```python
from build123d import *

# Parameters (mm, degrees)
DODANIE_WYCI_GNI_CIE1_DEPTH = 5
DODANIE_WYCI_GNI_CIE4_DEPTH = 8
DODANIE_WYCI_GNI_CIE5_DEPTH = 3
SZKIC8_R                    = 1.05
WYTNIJ_WYCI_GNI_CIE1_DEPTH  = 38.825793195
SZKIC9_R                    = 1.05
WYTNIJ_WYCI_GNI_CIE2_DEPTH  = 39.000906522
ZAOKR_GLENIE1_R             = 2.5
ZAOKR_GLENIE2_R             = 2.5
ZAOKR_GLENIE3_R             = 2
WYTNIJ_WYCI_GNI_CIE3_DEPTH  = 38.825793195


# Some blends are built 0.0001 mm under size
with BuildPart() as part:
    # Szkic1 → Dodanie-wyciągnięcie1 (new body)
    with BuildSketch(Plane.XY):
        Polygon((6.943729276, -9.167385079), (6.943729276, -12.167385079), (-29.356270724, -12.167385079), (-29.356270724, -9.167385079), (-26.62744343, -9.167385079), (-26.62744343, 10.832614921), (-23.706270724, 10.832614921), (-23.706270724, -9.167385079), (1.293729276, -9.167385079), (1.293729276, 10.832614921), (4.214901981, 10.832614921), (4.214901981, -9.167385079), align=None)
    extrude(amount=DODANIE_WYCI_GNI_CIE1_DEPTH)

    # Szkic5 → Dodanie-wyciągnięcie4 (add)
    with BuildSketch(Plane.XY.offset(5)):
        Polygon((-26.62744343, -9.167385079), (-23.706270724, -9.167385079), (1.293729276, -9.167385079), (4.214901981, -9.167385079), (6.943729276, -9.167385079), (6.943729276, -12.167385079), (-29.356270724, -12.167385079), (-29.356270724, -9.167385079), align=None)
    extrude(amount=DODANIE_WYCI_GNI_CIE4_DEPTH)

    # Szkic7 → Dodanie-wyciągnięcie5 (add)
    with BuildSketch(Plane(origin=(0, 0, 0), x_dir=(-1, 0, 0), z_dir=(0, 0, -1))):
        Polygon((-4.214901981, -9.167385079), (-1.293729276, -9.167385079), (23.706270724, -9.167385079), (26.62744343, -9.167385079), (29.356270724, -9.167385079), (29.356270724, -12.167385079), (-6.943729276, -12.167385079), (-6.943729276, -9.167385079), align=None)
    extrude(amount=DODANIE_WYCI_GNI_CIE5_DEPTH)

    # Szkic8 → Wytnij-wyciągnięcie1 (cut, through all)
    with BuildSketch(Plane(origin=(0, -9.167385079, 0), x_dir=(1, 0, 0), z_dir=(0, 1, 0))):
        with Locations(Location((4.446418634, -8, 0), (0, 0, 180))):
            Circle(SZKIC8_R)
        with Locations(Location((-26.853581366, -8, 0), (0, 0, 180))):
            Circle(SZKIC8_R)
    extrude(amount=-WYTNIJ_WYCI_GNI_CIE1_DEPTH, mode=Mode.SUBTRACT)

    # Szkic9 → Wytnij-wyciągnięcie2 (cut, through all)
    with BuildSketch(Plane.ZY.offset(26.62744343)):
        with Locations((2.5, 8.332614921)):
            Circle(SZKIC9_R)
    extrude(amount=-WYTNIJ_WYCI_GNI_CIE2_DEPTH, mode=Mode.SUBTRACT)

    # Zaokrąglenie1
    zaokr_glenie1_edges = [part.edges().sort_by_distance(p)[0] for p in [
        (-29.356270724, -10.667385079, 13),
        (6.943729276, -10.667385079, 13),
        (6.943729276, -10.667385079, -3),
        (-29.356270724, -10.667385079, -3),
    ]]
    fillet(zaokr_glenie1_edges, radius=ZAOKR_GLENIE1_R)

    # Zaokrąglenie2
    zaokr_glenie2_edges = [part.edges().sort_by_distance(p)[0] for p in [
        (-25.166857077, 10.832614921, 5),
        (-25.166857077, 10.832614921, 0),
        (2.754315628, 10.832614921, 5),
        (2.754315628, 10.832614921, 0),
    ]]
    fillet(zaokr_glenie2_edges, radius=ZAOKR_GLENIE2_R - 0.0001)  # a hair under: the kernel refuses the full size

    # Zaokrąglenie3
    # the kernel refuses this fillet: 2 mm, written as the material it adds along each edge
    with BuildSketch(Plane(origin=(4.214901981, -9.167385079, 0), x_dir=(1, 0, 0), z_dir=(0, 0, 1))) as zaokr_glenie3_piece_1:
        with BuildLine():
            CenterArc((ZAOKR_GLENIE3_R, ZAOKR_GLENIE3_R), ZAOKR_GLENIE3_R, 180, 90)
            Line((0, ZAOKR_GLENIE3_R), (0, 0))
            Line((0, 0), (ZAOKR_GLENIE3_R, 0))
        make_face()
    extrude(amount=5)
    with BuildSketch(Plane(origin=(-26.62744343, -9.167385079, 0), x_dir=(-1, 0, 0), z_dir=(0, 0, 1))) as zaokr_glenie3_piece_2:
        with BuildLine():
            CenterArc((ZAOKR_GLENIE3_R, -ZAOKR_GLENIE3_R), ZAOKR_GLENIE3_R, 90, 90)
            Line((0, -ZAOKR_GLENIE3_R), (0, 0))
            Line((0, 0), (ZAOKR_GLENIE3_R, 0))
        make_face()
    extrude(amount=5)
    with BuildSketch(Plane(origin=(-23.706270724, -9.167385079, 5), x_dir=(0, 1, 0), z_dir=(-1, 0, 0))) as zaokr_glenie3_piece_3_section:
        with BuildLine():
            CenterArc((ZAOKR_GLENIE3_R, -ZAOKR_GLENIE3_R), ZAOKR_GLENIE3_R, 90, 90)
            Line((0, -ZAOKR_GLENIE3_R), (0, 0))
            Line((0, 0), (ZAOKR_GLENIE3_R, 0))
        make_face()
    zaokr_glenie3_piece_3 = extrude(amount=2.921172706, mode=Mode.PRIVATE)
    zaokr_glenie3_piece_3 = zaokr_glenie3_piece_3 - Plane(origin=(-26.853581366, -8.714586813, 8), x_dir=(-1, 0, 0), z_dir=(0, 1, 0)) * Cylinder(1.05, 14, mode=Mode.PRIVATE)
    add(zaokr_glenie3_piece_3)
    with BuildSketch(Plane(origin=(4.214901981, -9.167385079, 5), x_dir=(0, 0, 1), z_dir=(-1, 0, 0))) as zaokr_glenie3_piece_4_section:
        with BuildLine():
            CenterArc((ZAOKR_GLENIE3_R, ZAOKR_GLENIE3_R), ZAOKR_GLENIE3_R, 180, 90)
            Line((0, ZAOKR_GLENIE3_R), (0, 0))
            Line((0, 0), (ZAOKR_GLENIE3_R, 0))
        make_face()
    zaokr_glenie3_piece_4 = extrude(amount=2.921172706, mode=Mode.PRIVATE)
    zaokr_glenie3_piece_4 = zaokr_glenie3_piece_4 - Plane(origin=(4.446418634, -8.714587659, 8), x_dir=(-1, 0, 0), z_dir=(0, 1, 0)) * Cylinder(1.05, 14, mode=Mode.PRIVATE)
    add(zaokr_glenie3_piece_4)
    with BuildSketch(Plane(origin=(1.293729276, -9.167385079, 0), x_dir=(0, 0, -1), z_dir=(1, 0, 0))) as zaokr_glenie3_piece_5:
        with BuildLine():
            CenterArc((ZAOKR_GLENIE3_R, ZAOKR_GLENIE3_R), ZAOKR_GLENIE3_R, 180, 90)
            Line((0, ZAOKR_GLENIE3_R), (0, 0))
            Line((0, 0), (ZAOKR_GLENIE3_R, 0))
        make_face()
    extrude(amount=2.921172706)
    with BuildSketch(Plane(origin=(-26.62744343, -9.167385079, 0), x_dir=(0, 1, 0), z_dir=(1, 0, 0))) as zaokr_glenie3_piece_6:
        with BuildLine():
            CenterArc((ZAOKR_GLENIE3_R, -ZAOKR_GLENIE3_R), ZAOKR_GLENIE3_R, 90, 90)
            Line((0, -ZAOKR_GLENIE3_R), (0, 0))
            Line((0, 0), (ZAOKR_GLENIE3_R, 0))
        make_face()
    extrude(amount=2.921172706)
    with BuildSketch(Plane(origin=(4.214901981, -9.167385079, -5), x_dir=(1, 0, 0), z_dir=(0, 0, 1))) as zaokr_glenie3_piece_7a_section:
        with BuildLine():
            CenterArc((ZAOKR_GLENIE3_R, ZAOKR_GLENIE3_R), ZAOKR_GLENIE3_R, 180, 90)
            Line((0, ZAOKR_GLENIE3_R), (0, 0))
            Line((0, 0), (ZAOKR_GLENIE3_R, 0))
        make_face()
    zaokr_glenie3_piece_7a = extrude(amount=10, mode=Mode.PRIVATE)
    zaokr_glenie3_piece_7a = zaokr_glenie3_piece_7a & Plane(origin=(4.443729276, -8.70886388, -0.5), x_dir=(1, 0, 0), z_dir=(0, 1, 0)) * Cylinder(2.5, 28, mode=Mode.PRIVATE)
    zaokr_glenie3_piece_7a = split(zaokr_glenie3_piece_7a, bisect_by=Plane(origin=(4.654982767, -8.70886388, 0), z_dir=(0, 0, -1)), keep=Keep.TOP, mode=Mode.PRIVATE)
    with BuildSketch(Plane(origin=(1.293729276, -9.167385079, 0), x_dir=(0, 0, -1), z_dir=(1, 0, 0))) as zaokr_glenie3_piece_7b_section:
        with BuildLine():
            CenterArc((ZAOKR_GLENIE3_R, ZAOKR_GLENIE3_R), ZAOKR_GLENIE3_R, 180, 90)
            Line((0, ZAOKR_GLENIE3_R), (0, 0))
            Line((0, 0), (ZAOKR_GLENIE3_R, 0))
        make_face()
    zaokr_glenie3_piece_7b = extrude(amount=7.921172706, mode=Mode.PRIVATE)
    zaokr_glenie3_piece_7b = zaokr_glenie3_piece_7b & Plane(origin=(4.443729276, -8.713013539, -0.5), x_dir=(1, 0, 0), z_dir=(0, 1, 0)) * Cylinder(2.5, 24, mode=Mode.PRIVATE)
    zaokr_glenie3_piece_7b = split(zaokr_glenie3_piece_7b, bisect_by=Plane(origin=(4.214901981, -8.713013539, -0.447003407), z_dir=(1, 0, 0)), keep=Keep.TOP, mode=Mode.PRIVATE)
    zaokr_glenie3_piece_7 = zaokr_glenie3_piece_7a & zaokr_glenie3_piece_7b
    add(zaokr_glenie3_piece_7)
    with BuildSketch(Plane(origin=(4.214901981, -9.167385079, 0), x_dir=(1, 0, 0), z_dir=(0, 0, 1))) as zaokr_glenie3_piece_8a_section:
        with BuildLine():
            CenterArc((ZAOKR_GLENIE3_R, ZAOKR_GLENIE3_R), ZAOKR_GLENIE3_R, 180, 90)
            Line((0, ZAOKR_GLENIE3_R), (0, 0))
            Line((0, 0), (ZAOKR_GLENIE3_R, 0))
        make_face()
    zaokr_glenie3_piece_8a = extrude(amount=10, mode=Mode.PRIVATE)
    zaokr_glenie3_piece_8a = zaokr_glenie3_piece_8a - Plane(origin=(4.446418634, -9.113524986, 8), x_dir=(-1, 0, 0), z_dir=(0, 1, 0)) * Cylinder(1.05, 28, mode=Mode.PRIVATE)
    zaokr_glenie3_piece_8a = split(zaokr_glenie3_piece_8a, bisect_by=Plane(origin=(5.693435365, -9.113524986, 5), z_dir=(0, 0, 1)), keep=Keep.TOP, mode=Mode.PRIVATE)
    with BuildSketch(Plane(origin=(9.214901981, -9.167385079, 5), x_dir=(0, 0, 1), z_dir=(-1, 0, 0))) as zaokr_glenie3_piece_8b_section:
        with BuildLine():
            CenterArc((ZAOKR_GLENIE3_R, ZAOKR_GLENIE3_R), ZAOKR_GLENIE3_R, 180, 90)
            Line((0, ZAOKR_GLENIE3_R), (0, 0))
            Line((0, 0), (ZAOKR_GLENIE3_R, 0))
        make_face()
    zaokr_glenie3_piece_8b = extrude(amount=7.921172706, mode=Mode.PRIVATE)
    zaokr_glenie3_piece_8b = split(zaokr_glenie3_piece_8b, bisect_by=Plane(origin=(6.943729276, -8.714456285, 5.452342783), z_dir=(-1, 0, 0)), keep=Keep.TOP, mode=Mode.PRIVATE)
    zaokr_glenie3_piece_8b = zaokr_glenie3_piece_8b - Plane(origin=(4.446418634, -8.714456285, 8), x_dir=(-1, 0, 0), z_dir=(0, 1, 0)) * Cylinder(1.05, 24, mode=Mode.PRIVATE)
    zaokr_glenie3_piece_8b = split(zaokr_glenie3_piece_8b, bisect_by=Plane(origin=(4.214901981, -8.714456285, 5.452342783), z_dir=(1, 0, 0)), keep=Keep.TOP, mode=Mode.PRIVATE)
    zaokr_glenie3_piece_8 = zaokr_glenie3_piece_8a & zaokr_glenie3_piece_8b
    add(zaokr_glenie3_piece_8)
    with BuildSketch(Plane(origin=(-31.62744343, -9.167385079, 0), x_dir=(0, 1, 0), z_dir=(1, 0, 0))) as zaokr_glenie3_piece_9a_section:
        with BuildLine():
            CenterArc((ZAOKR_GLENIE3_R, -ZAOKR_GLENIE3_R), ZAOKR_GLENIE3_R, 90, 90)
            Line((0, -ZAOKR_GLENIE3_R), (0, 0))
            Line((0, 0), (ZAOKR_GLENIE3_R, 0))
        make_face()
    zaokr_glenie3_piece_9a = extrude(amount=7.921172706, mode=Mode.PRIVATE)
    zaokr_glenie3_piece_9a = split(zaokr_glenie3_piece_9a, bisect_by=Plane(origin=(-26.62744343, -8.713013524, -0.447003529), z_dir=(-1, 0, 0)), keep=Keep.TOP, mode=Mode.PRIVATE)
    zaokr_glenie3_piece_9a = zaokr_glenie3_piece_9a & Plane(origin=(-26.856270724, -8.713013524, -0.5), x_dir=(0, 0, -1), z_dir=(0, -1, 0)) * Cylinder(2.5, 24, mode=Mode.PRIVATE)
    with BuildSketch(Plane(origin=(-26.62744343, -9.167385079, -5), x_dir=(-1, 0, 0), z_dir=(0, 0, 1))) as zaokr_glenie3_piece_9b_section:
        with BuildLine():
            CenterArc((ZAOKR_GLENIE3_R, -ZAOKR_GLENIE3_R), ZAOKR_GLENIE3_R, 90, 90)
            Line((0, -ZAOKR_GLENIE3_R), (0, 0))
            Line((0, 0), (ZAOKR_GLENIE3_R, 0))
        make_face()
    zaokr_glenie3_piece_9b = extrude(amount=10, mode=Mode.PRIVATE)
    zaokr_glenie3_piece_9b = split(zaokr_glenie3_piece_9b, bisect_by=Plane(origin=(-27.067524529, -8.708863922, 0), z_dir=(0, 0, -1)), keep=Keep.TOP, mode=Mode.PRIVATE)
    zaokr_glenie3_piece_9b = zaokr_glenie3_piece_9b & Plane(origin=(-26.856270724, -8.708863922, -0.5), x_dir=(0, 0, -1), z_dir=(0, -1, 0)) * Cylinder(2.5, 29, mode=Mode.PRIVATE)
    zaokr_glenie3_piece_9 = zaokr_glenie3_piece_9a & zaokr_glenie3_piece_9b
    add(zaokr_glenie3_piece_9)
    with BuildSketch(Plane(origin=(-23.706270724, -9.167385079, 5), x_dir=(0, 1, 0), z_dir=(-1, 0, 0))) as zaokr_glenie3_piece_10a_section:
        with BuildLine():
            CenterArc((ZAOKR_GLENIE3_R, -ZAOKR_GLENIE3_R), ZAOKR_GLENIE3_R, 90, 90)
            Line((0, -ZAOKR_GLENIE3_R), (0, 0))
            Line((0, 0), (ZAOKR_GLENIE3_R, 0))
        make_face()
    zaokr_glenie3_piece_10a = extrude(amount=7.921172706, mode=Mode.PRIVATE)
    zaokr_glenie3_piece_10a = split(zaokr_glenie3_piece_10a, bisect_by=Plane(origin=(-26.62744343, -8.714457191, 5.452345725), z_dir=(-1, 0, 0)), keep=Keep.TOP, mode=Mode.PRIVATE)
    zaokr_glenie3_piece_10a = split(zaokr_glenie3_piece_10a, bisect_by=Plane(origin=(-29.356270724, -8.714457191, 5.452345725), z_dir=(1, 0, 0)), keep=Keep.TOP, mode=Mode.PRIVATE)
    zaokr_glenie3_piece_10a = zaokr_glenie3_piece_10a - Plane(origin=(-26.853581366, -8.714457191, 8), x_dir=(-1, 0, 0), z_dir=(0, 1, 0)) * Cylinder(1.05, 24, mode=Mode.PRIVATE)
    with BuildSketch(Plane(origin=(-26.62744343, -9.167385079, 0), x_dir=(-1, 0, 0), z_dir=(0, 0, 1))) as zaokr_glenie3_piece_10b_section:
        with BuildLine():
            CenterArc((ZAOKR_GLENIE3_R, -ZAOKR_GLENIE3_R), ZAOKR_GLENIE3_R, 90, 90)
            Line((0, -ZAOKR_GLENIE3_R), (0, 0))
            Line((0, 0), (ZAOKR_GLENIE3_R, 0))
        make_face()
    zaokr_glenie3_piece_10b = extrude(amount=10, mode=Mode.PRIVATE)
    zaokr_glenie3_piece_10b = split(zaokr_glenie3_piece_10b, bisect_by=Plane(origin=(-28.105975739, -9.113528996, 5), z_dir=(0, 0, 1)), keep=Keep.TOP, mode=Mode.PRIVATE)
    zaokr_glenie3_piece_10b = zaokr_glenie3_piece_10b - Plane(origin=(-26.853581366, -9.113528996, 8), x_dir=(-1, 0, 0), z_dir=(0, 1, 0)) * Cylinder(1.05, 29, mode=Mode.PRIVATE)
    zaokr_glenie3_piece_10 = zaokr_glenie3_piece_10a & zaokr_glenie3_piece_10b
    add(zaokr_glenie3_piece_10)

    # Szkic10 → Wytnij-wyciągnięcie3 (cut, through all)
    with BuildSketch(Plane(origin=(0, -9.167385079, 0), x_dir=(1, 0, 0), z_dir=(0, 1, 0))):
        with BuildLine():
            Line((-18.706270724, -8), (-3.706270724, -8))
            ThreePointArc((-3.706270724, -8), (-0.706270724, -5), (-3.706270724, -2))
            Line((-3.706270724, -2), (-18.706270724, -2))
            ThreePointArc((-18.706270724, -2), (-21.706270724, -5), (-18.706270724, -8))
        make_face()
    extrude(amount=-WYTNIJ_WYCI_GNI_CIE3_DEPTH, mode=Mode.SUBTRACT)


solid = part.part
```
Work out the finished part from the listing and answer in its coordinate system (mm). A direction names the side the tool comes from. Round coordinates to 2 decimals unless told otherwise and drop trailing zeros. Loops run counter-clockwise (first coordinate to the right, second up) from the corner with the lowest first, then second, coordinate; pieces in that order, holes last. Notation, with made-up numbers: (-16, 54.25) -> (28, 54.25) arc R28 cw to (28, 78.25) -> close; hole circle Ø4 at (81.5, 54.25). An arc over 180 degrees is marked (long way). Write each question's results on one line, items separated by ' | '. Start each with the question number.
1. Given pin 1 Ø1.5 at (y, z) = (2, 1.5) entering from -X; pin 2 Ø2.5 at (y, z) = (-2.5, 3.5) entering from +X; pin 3 Ø1.5 at (x, y) = (2.5, 3) entering from -Z, each flat-ended and moving along its own axis, determine where each tip first touches the part or whether it passes through.
2. Section D-D (y = -9.75) is taken. Determine the outline of the cut face in (x, z).
3. Find the intervals of material crossed by probe 1 along Z at (x, y) = (-10, -9.5); probe 2 along X at (y, z) = (4.75, 4.25); probe 3 along Y at (x, z) = (-24.9, 2.5), in increasing order. Write a range as from..to.
4. A tool of negligible diameter and unlimited length cuts with its end or side. For faces 4 (the face through (-11, -11, 8)), 5 (the face through (1.294, 1, 2)), 6 (the face through (3, 1, 0)), from which of +Z, -Z, +X, -X, +Y, -Y can it reach the whole face along a straight path? Write none if from no direction.
5. Section A-A (y = 3.25) is taken. Determine the outline of the cut face in (x, z), plus the area to 3 significant figures.
6. For a pull along Y with two mould halves and no side action, classify faces 1 (the face through (2.73, 8.65, 3.5)), 2 (the face through (2.77, 10.08, 0.71)), 3 (the face through (-29.356, -11, 5)) as +Y half, -Y half, draft (parallel to the pull), parting line (faces both ways), or undercut.
7. Section C-C (z = 8.5) is taken. Determine the outline of the cut face in (x, y).
8. Section B-B (x = -11) is taken. Determine the outline of the cut face in (y, z).
Evaluation:
1) pin 1: stops at x = -26.63 | pin 2: stops at x = 4.21 | pin 3: stops at z = 0
2) outline: (-29.36, -0.5) arc R2.5 ccw to (-26.86, -3) -> (4.44, -3) arc R2.5 ccw to (6.94, -0.5) -> (6.94, 10.5) arc R2.5 ccw to (4.44, 13) -> (-26.86, 13) arc R2.5 ccw to (-29.36, 10.5) -> close; hole circle Ø2.1 at (-26.85, 8); hole (-18.71, 2) -> (-3.71, 2) arc R3 ccw to (-3.71, 8) -> (-18.71, 8) arc R3 ccw to start; hole circle Ø2.1 at (4.45, 8)
3) probe 1: z = -3..2, 8..13 | probe 2: x = -26.63..-23.71, 1.29..4.21 | probe 3: y = -12.17..7.28, 9.38..10.83
4) face 4: +Y, -Y | face 5: +Z, -Z, +Y | face 6: -Z, +X, -X, +Y
5) outline: (-26.63, 0) -> (-23.71, 0) -> (-23.71, 5) -> (-26.63, 5) -> close; (1.29, 0) -> (4.21, 0) -> (4.21, 5) -> (1.29, 5) -> close | area: 29.2 mm2
6) face 1: undercut | face 2: +Y half | face 3: draft
7) outline: (-29.36, -12.17) -> (-27.78, -12.17) -> (-27.78, -9.17) -> (-29.36, -9.17) -> close; (-25.93, -12.17) -> (3.52, -12.17) -> (3.52, -9.17) -> (-25.93, -9.17) -> close; (5.37, -12.17) -> (6.94, -12.17) -> (6.94, -9.17) -> (5.37, -9.17) -> close
8) outline: (-12.17, -3) -> (-9.17, -3) -> (-9.17, 2) -> (-12.17, 2) -> close; (-12.17, 8) -> (-9.17, 8) -> (-9.17, 13) -> (-12.17, 13) -> close
